Source: CAD feature listing. Evaluate the final solid. Frame: model axes, mm. A direction names the side the tool comes from. Coordinates: 2 decimals unless noted, no trailing zeros. Write each loop counter-clockwise with the first axis right and the second up, starting at its lowest first coordinate (ties: lowest second). Pieces come first, ordered by that corner, then holes. Notation, with made-up numbers: M 67,-27 L 91,-27 A15 ccw 91,-13 Z; hole C 6,67 d8. An arc over 180 degrees is marked long. Write item = value, one per line. Start each with the question number.
1. Line query: line 1 along Z through (x, y) = (0, 23); line 2 along Z through (x, y) = (0, 4.5); line 3 along Z through (x, y) = (8, 12). Output: solid intervals per line, ascending.
2. Section query A-A (z = 25.4). Output: boundary loops of the cut face in (x, y).
3. Access query for faces 3 (the face through (21.844, 14.9, 5.3)), 4 (the face through (-9.08, 13.5, 0.88)), 5 (the face through (6, 2.032, 6)), 6 (the face through (0.83, 2.41, -3.72)). Directions: +Z, -Z, +X, -X, +Y, -Y. A direction counts if a zero-diameter tool reaches every point of the face in a straight line with its end or side. Return the directions, or none.
4. Pull-direction query (Z, two-part tool) for faces 1 (the face through (14, -6.35, 0)), 2 (the face through (18.338, 7.185, 0.724)); classes: pulls with the +Z half, pulls with the -Z half, needs draft (parallel to the pull), parting line crosses it, or undercut.
5. Pin query (flat end, axial travel): pin 1 Ø3.5 at (y, z) = (14, 0.5) entering from +X; pin 2 Ø3 at (y, z) = (18.5, 1) entering from +X; pin 3 Ø8 at (y, z) = (-1, -18) entering from -X; pin 4 Ø2.5 at (y, z) = (12.7, 0) entering from -X. Return the tip coordinate at first contact, or that it passes through.
6. Section query C-C (x = 0). Give the number of separate pieces and of enclosed holes in the cut face, then the cut area to 3 significant figures.
7. Section query B-B (x = 24.5). Output: boundary loops of the cut face in (y, z), then the cut area to 3 significant figures.
```python
from build123d import *

# Parameters (mm, degrees)
M14X1_5_TAPPED_HOLE1_D              = 12.5
M14X1_5_TAPPED_HOLE1_DEPTH          = 25.4
M14X1_5_TAPPED_HOLE1_TIP            = 3.755378869
F_1_16_0_0625_DIAMETER_HOLE1_D      = 1.5875
F_1_16_0_0625_DIAMETER_HOLE1_DEPTH  = 28.575
F_1_16_0_0625_DIAMETER_HOLE1_TIP    = 0.476933116
F_3_32_0_09375_DIAMETER_HOLE1_D     = 2.38125
F_3_32_0_09375_DIAMETER_HOLE1_DEPTH = 28.702
F_3_32_0_09375_DIAMETER_HOLE1_TIP   = 0.715399675
F_1_4_CLEARANCE_HOLE1_D             = 6.7564
CIRPATTERN1_COUNT                   = 6
F_1_32_0_03125_DIAMETER_HOLE1_D     = 0.79375
F_1_32_0_03125_DIAMETER_HOLE1_DEPTH = 28.575
F_1_32_0_03125_DIAMETER_HOLE1_TIP   = 0.238466558


with BuildPart() as part:
    # Sketch1 → Revolve1 (revolve)
    with BuildSketch(Plane.XY):
        Polygon((-3.81, 0), (-8.0645, 0), (-8.0645, 2.032), (-11.1125, 2.032), (-11.1125, 0), (-12.7, 0), (-12.7, -6.35), (-31.75, -6.35), (-31.75, 31.75), (-3.81, 31.75), align=None)
    revolve(axis=Axis((0, 0, 0), (0, 1, 0)))

    # M14x1.5 Tapped Hole1
    with Locations(Plane(origin=(0, 31.75, 0), x_dir=(1, 0, 0), z_dir=(0, 1, 0))):
        with Locations((0, 0)):
            Hole(M14X1_5_TAPPED_HOLE1_D / 2, depth=M14X1_5_TAPPED_HOLE1_DEPTH)
            with Locations((0, 0, -(M14X1_5_TAPPED_HOLE1_DEPTH + M14X1_5_TAPPED_HOLE1_TIP / 2))):  # 118° drill point
                Cone(0, M14X1_5_TAPPED_HOLE1_D / 2, M14X1_5_TAPPED_HOLE1_TIP, mode=Mode.SUBTRACT)

    # Sketch6 → 1/4 NPT Tapped Hole1 (revolve, cut)
    with BuildSketch(Plane(origin=(31.75, 12.7, 0), x_dir=(0, 0, -1), z_dir=(0, 1, 0))):
        Polygon((0, 0), (0, 20.360347279), (5.5626, 17.018), (5.5626, 9.906), (5.943685794, 9.906), (6.2402847, 0), align=None)
    revolve(axis=Axis((38.1, 12.7, 0), (-1, 0, 0)), mode=Mode.SUBTRACT)

    # Sketch8 → 1/4 NPT Tapped Hole2 (revolve, cut)
    with BuildSketch(Plane(origin=(-31.75, 12.7, 0), x_dir=(0, 0, 1), z_dir=(0, 1, 0))):
        Polygon((0, 0), (0, 20.360347279), (5.5626, 17.018), (5.5626, 9.906), (5.943685794, 9.906), (6.2402847, 0), align=None)
    revolve(axis=Axis((-38.1, 12.7, 0), (1, 0, 0)), mode=Mode.SUBTRACT)

    # 1/16 (0.0625) Diameter Hole1
    with Locations(Plane(origin=(31.75, 0, 0), x_dir=(0, 0, -1), z_dir=(1, 0, 0))):
        with Locations((0, 12.7)):
            Hole(F_1_16_0_0625_DIAMETER_HOLE1_D / 2, depth=F_1_16_0_0625_DIAMETER_HOLE1_DEPTH)
            with Locations((0, 0, -(F_1_16_0_0625_DIAMETER_HOLE1_DEPTH + F_1_16_0_0625_DIAMETER_HOLE1_TIP / 2))):  # 118° drill point
                Cone(0, F_1_16_0_0625_DIAMETER_HOLE1_D / 2, F_1_16_0_0625_DIAMETER_HOLE1_TIP, mode=Mode.SUBTRACT)

    # 3/32 (0.09375) Diameter Hole1
    with Locations(Plane.ZY.offset(31.75)):
        with Locations((0, 12.7)):
            Hole(F_3_32_0_09375_DIAMETER_HOLE1_D / 2, depth=F_3_32_0_09375_DIAMETER_HOLE1_DEPTH)
            with Locations((0, 0, -(F_3_32_0_09375_DIAMETER_HOLE1_DEPTH + F_3_32_0_09375_DIAMETER_HOLE1_TIP / 2))):  # 118° drill point
                Cone(0, F_3_32_0_09375_DIAMETER_HOLE1_D / 2, F_3_32_0_09375_DIAMETER_HOLE1_TIP, mode=Mode.SUBTRACT)

    # 1/4 Clearance Hole1 (through all)
    with Locations(Plane(origin=(0, 31.75, 0), x_dir=(1, 0, 0), z_dir=(0, 1, 0))):
        with Locations((21.997045256, 12.7)):
            f_1_4_clearance_hole1 = Hole(F_1_4_CLEARANCE_HOLE1_D / 2)

    # CirPattern1: 1/4 Clearance Hole1 ×6 about axis
    cirpattern1_axis = Axis((0, 0, 0), (0, 1, 0))
    for i in range(1, CIRPATTERN1_COUNT):
        add(f_1_4_clearance_hole1.rotate(cirpattern1_axis, i * 360 / CIRPATTERN1_COUNT), mode=Mode.SUBTRACT)

    # Sketch18 → 1/4 NPT Tapped Hole3 (revolve, cut)
    with BuildSketch(Plane(origin=(15.875, 12.7, -27.49630657), x_dir=(-0.866025404, 0, -0.5), z_dir=(0, 1, 0))):
        Polygon((0, 0), (0, 19.852347279), (5.5626, 16.51), (5.5626, 12.7), (6.557983593, 12.7), (6.9382386, 0), align=None)
    revolve(axis=Axis((19.05, 12.7, -32.995567884), (-0.5, 0, 0.866025404)), mode=Mode.SUBTRACT)

    # 1/32 (0.03125) Diameter Hole1
    with Locations(Plane(origin=(15.875, 0, -27.49630657), x_dir=(0, -1, 0), z_dir=(0.5, 0, -0.866025404))):
        with Locations((-12.7, 0)):
            Hole(F_1_32_0_03125_DIAMETER_HOLE1_D / 2, depth=F_1_32_0_03125_DIAMETER_HOLE1_DEPTH)
            with Locations((0, 0, -(F_1_32_0_03125_DIAMETER_HOLE1_DEPTH + F_1_32_0_03125_DIAMETER_HOLE1_TIP / 2))):  # 118° drill point
                Cone(0, F_1_32_0_03125_DIAMETER_HOLE1_D / 2, F_1_32_0_03125_DIAMETER_HOLE1_TIP, mode=Mode.SUBTRACT)


solid = part.part
```
Results are:
q1.line_1 = -31.75 to -28.78, -22.02 to -6.25, 6.25 to 22.02, 28.78 to 31.75
q1.line_2 = -31.75 to -28.78, -22.02 to -3.81, 3.81 to 22.02, 28.78 to 31.75
q1.line_3 = -30.73 to -27.42, -10.41 to -0.37, 0.37 to 30.73
q2.outline = M -19.05,-6.35 L -3.38,-6.35 L -3.38,31.75 L -19.05,31.75 Z; M 3.38,-6.35 L 19.05,-6.35 L 19.05,31.75 L 3.38,31.75 Z
q3.face_3 = +X
q3.face_4 = -X
q3.face_5 = -Y
q3.face_6 = +Y, -Y
q4.face_1 = needs draft
q4.face_2 = undercut
q5.pin_1 = 13.28
q5.pin_2 = 31.75
q5.pin_3 = -28.5
q5.pin_4 = -12.14
q6.separate_pieces = 4
q6.enclosed_holes = 0
q6.area = 1,360 mm^2
q7.outline = M -6.35,-20.19 L 31.75,-20.19 L 31.75,-14.97 L -6.35,-14.97 Z; M -6.35,-10.43 L 31.75,-10.43 L 31.75,10.43 L -6.35,10.43 Z; M -6.35,14.97 L 31.75,14.97 L 31.75,20.19 L -6.35,20.19 Z; hole C 12.7,0 d12.05
q7.area = 1,080 mm^2
